The model under review builds one solid part; all positions refer to its coordinate system, in mm. Face numbers are marked on the shaded views. A direction names the side the tool comes from. Round coordinates to 2 decimals unless told otherwise and drop trailing zeros. Order: outer loops, then holes, each group sorted by start corner. A loop starts at its lowest first (then second) coordinate and runs counter-clockwise, first axis right, second up. Notation, with made-up numbers: (71, 6.25) -> (93, 6.25) arc R32 cw to (93, 35.25) -> close; hole circle Ø3 at (5.5, 3). An arc over 180 degrees is marked (long way). Use a Markdown table: item, result. Add a question column.
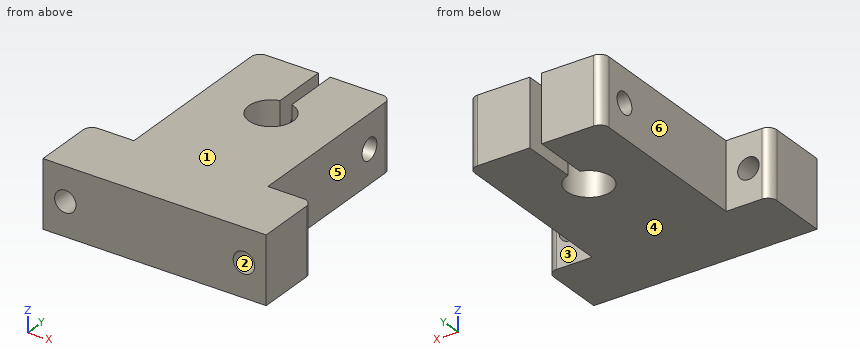
```python
from build123d import *

# Parameters (mm, degrees)
SKETCH1_W                       = 50
SKETCH1_H                       = 15
SKETCH1_R                       = 2.4
BOSS_EXTRUDE1_DEPTH             = 15
BOSS_EXTRUDE2_REACH             = 32.104
BOSS_EXTRUDE2_DIRECTION_2_REACH = 32.104
FILLET1_R                       = 2
SKETCH4_R                       = 2.4
CUT_EXTRUDE1_DEPTH              = 69.419660917


with BuildPart() as part:
    # Sketch1 → Boss-Extrude1 (new body)
    with BuildSketch(Plane(origin=(0, 0, 0), x_dir=(1, 0, 0), z_dir=(0, 1, 0))):
        Rectangle(SKETCH1_W, SKETCH1_H)
        with Locations(Location((-20, 0, 0), (0, 0, 270))):
            Circle(SKETCH1_R, mode=Mode.SUBTRACT)
        with Locations(Location((20, 0, 0), (0, 0, 90))):
            Circle(SKETCH1_R, mode=Mode.SUBTRACT)
    extrude(amount=BOSS_EXTRUDE1_DEPTH)

    # Boss-Extrude2: up to this face of the body (flat: up to its plane)
    boss_extrude2_end = Plane(part.part.faces().sort_by_distance((0, 7.5, 7.5))[0])
    # Sketch3 → Boss-Extrude2 (add, up to the picked face)
    with BuildSketch(Plane.XY, mode=Mode.PRIVATE) as boss_extrude2_sk1:
        with BuildLine():
            Line((1.328723236, 55), (1.328723236, 42.566882454))
            ThreePointArc((1.328723236, 42.566882454), (0, 32.746665181), (-1.328723236, 42.566882454))
            Line((-1.328723236, 42.566882454), (-1.328723236, 55))
            Line((-1.328723236, 55), (-3.865793159, 55))
            Line((-3.865793159, 55), (-13, 55))
            ThreePointArc((-13, 55), (-14.414213562, 54.414213562), (-15, 53))
            Line((-15, 53), (-15, 15))
            Line((-15, 15), (15, 15))
            Line((15, 15), (15, 53))
            ThreePointArc((15, 53), (14.414213562, 54.414213562), (13, 55))
            Line((13, 55), (3.865793159, 55))
            Line((3.865793159, 55), (1.328723236, 55))
        make_face()
    boss_extrude2_tool1 = split(extrude(boss_extrude2_sk1.sketch, amount=BOSS_EXTRUDE2_REACH, mode=Mode.PRIVATE), bisect_by=boss_extrude2_end, keep=Keep.BOTH, mode=Mode.PRIVATE)
    add(boss_extrude2_tool1.solids().sort_by(Axis((14.06066, 54.06066, 0), (0, 0, 1)))[0])

    # Boss-Extrude2 direction 2: up to this face of the body (flat: up to its plane)
    boss_extrude2_direction_2_end = Plane(part.part.faces().sort_by_distance((0, 7.5, -7.5))[0])
    # Sketch3 → Boss-Extrude2 direction 2 (add, up to the picked face)
    with BuildSketch(Plane.XY, mode=Mode.PRIVATE) as boss_extrude2_direction_2_sk1:
        with BuildLine():
            Line((1.328723236, 55), (1.328723236, 42.566882454))
            ThreePointArc((1.328723236, 42.566882454), (0, 32.746665181), (-1.328723236, 42.566882454))
            Line((-1.328723236, 42.566882454), (-1.328723236, 55))
            Line((-1.328723236, 55), (-3.865793159, 55))
            Line((-3.865793159, 55), (-13, 55))
            ThreePointArc((-13, 55), (-14.414213562, 54.414213562), (-15, 53))
            Line((-15, 53), (-15, 15))
            Line((-15, 15), (15, 15))
            Line((15, 15), (15, 53))
            ThreePointArc((15, 53), (14.414213562, 54.414213562), (13, 55))
            Line((13, 55), (3.865793159, 55))
            Line((3.865793159, 55), (1.328723236, 55))
        make_face()
    boss_extrude2_direction_2_tool1 = split(extrude(boss_extrude2_direction_2_sk1.sketch, amount=-BOSS_EXTRUDE2_DIRECTION_2_REACH, mode=Mode.PRIVATE), bisect_by=boss_extrude2_direction_2_end, keep=Keep.BOTH, mode=Mode.PRIVATE)
    add(boss_extrude2_direction_2_tool1.solids().sort_by(Axis((14.06066, 54.06066, 0), (0, 0, -1)))[0])

    # Fillet1
    fillet1_edges = [part.edges().sort_by_distance(p)[0] for p in [
        (25, 15, 0),
        (-25, 15, 0),
    ]]
    fillet(fillet1_edges, radius=FILLET1_R)

    # Sketch4 → Cut-Extrude1 (cut, through all)
    with BuildSketch(Plane.ZY.offset(15)):
        with Locations((0, 47.934840873)):
            Circle(SKETCH4_R)
    extrude(amount=-CUT_EXTRUDE1_DEPTH, mode=Mode.SUBTRACT)


solid = part.part
```
Q1. Mouldability with a two-part tool opening along Z and no side actions: class the marked faces 1, 2 and 3 as pulls with the +Z half, pulls with the -Z half, needs draft (parallel to the pull), parting line crosses it, or undercut.
Q2. Add section B-B (z = 0). State how many separate pieces and enclosed holes the cut face has, then the cut area to 3 significant figures.
Q3. Add section A-A (x = 20). Write out the cut boundary in (y, z), then the cut area to 3 significant figures.
Q4. Insertion check: pin 1 (6 mm diameter, centred on x = -20, z = 0, fed in from +Y); pin 2 (2 mm diameter, centred on y = 38, z = 0, fed in from -X); pin 3 (3.5 mm diameter, centred on y = 46.5, z = -3.5, fed in from +X). Each pin has a flat end and moves straight along its axis. Give the tip position at first contact, or say it passes through.
Q5. Add section D-D (y = 6.5). Write out the cut boundary in (x, z).
Q6. Wall thickness on line 1 (X direction, y = 8.5, z = -0.25); line 2 (Y direction, x = 5.5, z = 0); line 3 (X direction, y = 48, z = -5): over which ranges is each line inside the solid? List them lowest first. Write a range as [from, to].
Q7. Machinability: for the marked faces 4, 5 and 6, which of the approach directions +Z, -Z, +X, -X, +Y, -Y give a long, thin tool a straight path to every point of the face, cutting with its end or side? Answer none if there is none.
Q8. Add section C-C (z = -6.5). Write out the cut boundary in (x, y), then the cut area to 3 significant figures.
Report:
| question | item | result |
|---|---|---|
| 1 | face 1 | pulls with the +Z half |
| 1 | face 2 | undercut |
| 1 | face 3 | needs draft |
| 2 | separate pieces | 5 |
| 2 | enclosed holes | 0 |
| 2 | area | 1,560 mm² |
| 3 | outline | (0, -7.5) -> (15, -7.5) -> (15, -2.4) -> (0, -2.4) -> close; (0, 2.4) -> (15, 2.4) -> (15, 7.5) -> (0, 7.5) -> close |
| 3 | area | 153 mm² |
| 4 | pin 1 | stops at y = 15 |
| 4 | pin 2 | stops at x = -15 |
| 4 | pin 3 | stops at x = 15 |
| 5 | outline | (-25, -7.5) -> (25, -7.5) -> (25, 7.5) -> (-25, 7.5) -> close; hole circle Ø4.8 at (-20, 0); hole circle Ø4.8 at (20, 0) |
| 6 | line 1 | x = [-25, -22.39], [-17.61, 17.61], [22.39, 25] |
| 6 | line 2 | y = [0, 45.53], [50.33, 55] |
| 6 | line 3 | x = [-15, -1.33], [1.33, 15] |
| 7 | face 4 | -Z, +X, -X, +Y, -Y |
| 7 | face 5 | +Z, -Z, +X, +Y |
| 7 | face 6 | +Z, -Z, -X, +Y |
| 8 | outline | (-25, 0) -> (25, 0) -> (25, 13) arc R2 ccw to (23, 15) -> (15, 15) -> (15, 53) arc R2 ccw to (13, 55) -> (1.33, 55) -> (1.33, 42.57) arc R5 cw (long way) to (-1.33, 42.57) -> (-1.33, 55) -> (-13, 55) arc R2 ccw to (-15, 53) -> (-15, 15) -> (-23, 15) arc R2 ccw to (-25, 13) -> close |
| 8 | area | 1,840 mm² |
